from build123d import *

# Parameters (mm, degrees)
F1_DEPTH = 57
F2_R     = 1.75
F3_DEPTH = 10
F4_R     = 1.725
F5_DEPTH = 4


with BuildPart() as f1:
    # F0 (on Top) → F1 (new body)
    with BuildSketch(Plane.XY):
        Polygon((2.375, 1.371207), (0, 2.742414), (-2.375, 1.371207), (-2.375, -1.371207), (0, -2.742414), (2.375, -1.371207), align=None)
    extrude(amount=F1_DEPTH)

    # F2 (on face) → F3 (cut)
    with BuildSketch(Plane.XY.offset(57)):
        Circle(F2_R)
    extrude(amount=-F3_DEPTH, mode=Mode.SUBTRACT)

    # F4 (on face) → F5 (join)
    with BuildSketch(Plane(origin=(0, 0, 0), x_dir=(1, 0, 0), z_dir=(0, 0, -1))):
        Circle(F4_R)
    extrude(amount=F5_DEPTH)


solid = f1.part
Source: CAD feature listing. Evaluate the final solid. Frame: model axes, mm. A direction names the side the tool comes from. Round coordinates to 2 decimals unless told otherwise and drop trailing zeros. Loops run counter-clockwise (first coordinate to the right, second up) from the corner with the lowest first, then second, coordinate; pieces in that order, holes last.
Q1. Access query for faces 1 (the face through (0, -2, 0)), 2 (the face through (0, 0, 47)), 3 (the face through (-2.375, 0, 28)). Directions: +Z, -Z, +X, -X, +Y, -Y. A direction counts if a zero-diameter tool reaches every point of the face in a straight line with its end or side. Return the directions, or none.
Q2. Ray query, line 1 (Y direction, x = 0, z = 50); line 2 (Z direction, x = 2, y = -1.2); line 3 (Z direction, x = 0.85, y = 0.1). Return the intervals inside material, ascending.
Q3. Section A-A, the plane z = 52.5. Return loops of the section in (x, y) (3 decimals).
Q4. Mould query, pull axis Y, two halves, no side actions, for faces 4 (the face through (1.617, -0.67, 52.07)), 5 (the face through (1.171, -2.066, 28.101)), 6 (the face through (-1.171, 2.066, 28.101)). Classes: pulls with the +Y half, pulls with the -Y half, needs draft (parallel to the pull), parting line crosses it, or undercut.
Q5. Section C-C, the plane x = -1.1. Return loops of the section in (y, z), plus the area to 3 significant figures.
Q6. First-contact query: P1, Ø1, axis at x = 0, y = 0, coming from the +Z side; P2, Ø1.5, axis at x = 1.5, z = 43.5, coming from the +Y side. Flat tips, straight axial feed; report the tip coordinate or a pass-through.
Q7. Section B-B, the plane y = 0. Return loops of the section in (x, z) (3 decimals), plus the area to 3 significant figures.
Solutions:
1. face 1: -Z
1. face 2: +Z
1. face 3: +Z, -Z, -X, +Y, -Y
2. line 1: y = -2.74 to -1.75, 1.75 to 2.74
2. line 2: z = 0 to 57
2. line 3: z = -4 to 47
3. outline: (-2.375, -1.371) - (0, -2.742) - (2.375, -1.371) - (2.375, 1.371) - (0, 2.742) - (-2.375, 1.371) - close; hole circle Ø3.5 at (0, 0)
4. face 4: undercut
4. face 5: pulls with the -Y half
4. face 6: pulls with the +Y half
5. outline: (-2.11, 0) - (-1.33, 0) - (-1.33, -4) - (1.33, -4) - (1.33, 0) - (2.11, 0) - (2.11, 57) - (1.36, 57) - (1.36, 47) - (-1.36, 47) - (-1.36, 57) - (-2.11, 57) - close
5. area: 224 mm2
6. P1: stops at z = 47
6. P2: stops at y = 2.31
7. outline: (-2.375, 0) - (-1.725, 0) - (-1.725, -4) - (1.725, -4) - (1.725, 0) - (2.375, 0) - (2.375, 57) - (1.75, 57) - (1.75, 47) - (-1.75, 47) - (-1.75, 57) - (-2.375, 57) - close
7. area: 250 mm2
